Input: dimensioned drawing with shaded views. Units: mm. Origin: part minimum x, y, z. A direction names the side the tool comes from. Give positions to 0.01 mm unless a question says otherwise; leave off trailing zeros. Write each loop counter-clockwise with the first axis right and the second up, starting at its lowest first coordinate (ties: lowest second). Pieces come first, ordered by that corner, then holes. Notation, with made-up numbers: (9.5, -24.5) -> (58.5, -24.5) arc R33 ccw to (58.5, 14.5) -> close; hole circle Ø5 at (30.25, 86.25). An arc over 180 degrees is marked (long way). Return JSON: item names as keys, results as strings. Group by question number.
Item 1: Section C-C, the plane z = 10.5. Return loops of the section in (x, y).
Item 2: Set-up query: the marked faces 1 and 2. Return all of +Z, -Z, +X, -X, +Y, -Y with unobstructed straight access to the full face (end or side cutting, diameter ignored); none if empty.
Item 3: Section D-D, the plane x = 51.5. Return loops of the section in (y, z).
Item 4: Pin query (flat end, axial travel): P1, Ø3.5, axis at x = 12.4, z = 32.6, coming from the -Y side; P2, Ø1.5, axis at x = 45, y = 1.5, coming from the +Z side; P3, Ø0.9, axis at x = 3.5, y = 13.5, coming from the -Z side. Return the tip coordinate at first contact, or that it passes through.
Item 5: Line query: line 1 (X direction, y = 13.8, z = 10.5); line 2 (X direction, y = 14.2, z = 32.6); line 3 (Y direction, x = 31, z = 21). Output: solid intervals per line, ascending. Write a range as [from, to].
Item 6: Section B-B, the plane y = 7.25. Return loops of the section in (x, z), then the cut area to 3 significant figures.
Item 7: Section A-A, the plane x = 12.4. Return loops of the section in (y, z).
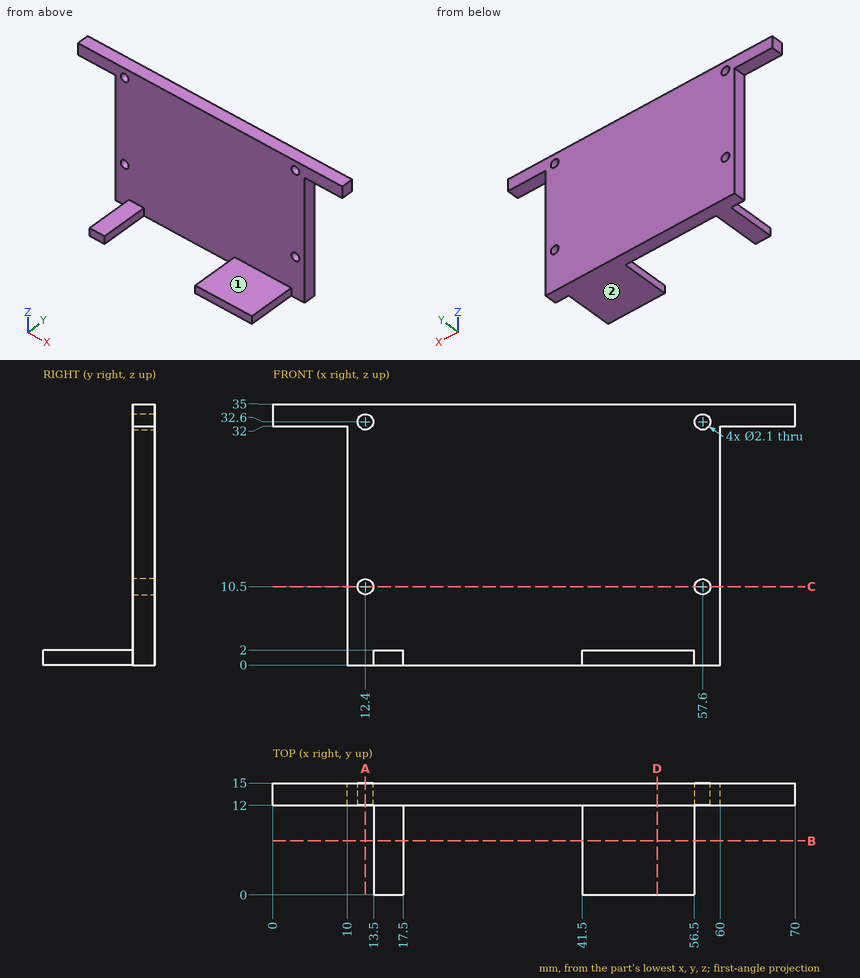
Answer below:
{
 "1": {"outline": "(10, 12) -> (11.35, 12) -> (11.35, 15) -> (10, 15) -> close; (13.45, 12) -> (56.55, 12) -> (56.55, 15) -> (13.45, 15) -> close; (58.65, 12) -> (60, 12) -> (60, 15) -> (58.65, 15) -> close"},
 "2": {"face 1": "+Z, +X, -X, -Y", "face 2": "-Z, +X, -X, +Y, -Y"},
 "3": {"outline": "(0, 0) -> (15, 0) -> (15, 35) -> (12, 35) -> (12, 2) -> (0, 2) -> close"},
 "4": {"P1": "stops at y = 12", "P2": "stops at z = 2", "P3": "stops at z = 32"},
 "5": {"line 1": "x = [10, 11.35], [13.45, 56.55], [58.65, 60]", "line 2": "x = [0, 11.35], [13.45, 56.55], [58.65, 70]", "line 3": "y = [12, 15]"},
 "6": {"outline": "(13.5, 0) -> (17.5, 0) -> (17.5, 2) -> (13.5, 2) -> close; (41.5, 0) -> (56.5, 0) -> (56.5, 2) -> (41.5, 2) -> close", "area": "38.0 mm2"},
 "7": {"outline": "(12, 0) -> (15, 0) -> (15, 9.45) -> (12, 9.45) -> close; (12, 11.55) -> (15, 11.55) -> (15, 31.55) -> (12, 31.55) -> close; (12, 33.65) -> (15, 33.65) -> (15, 35) -> (12, 35) -> close"}
}
